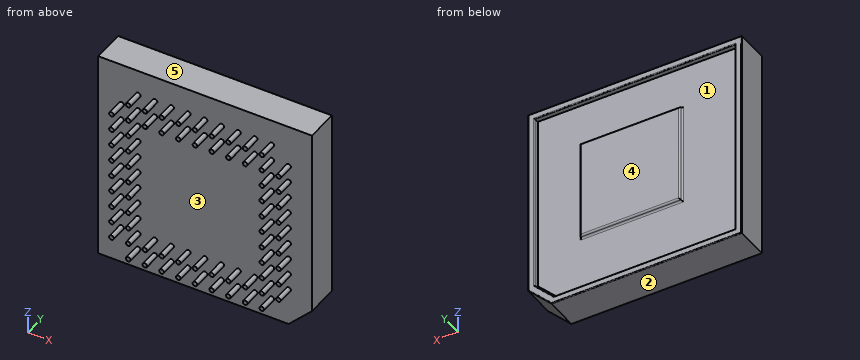
from build123d import *

# Parameters (mm, degrees)
BASE_EXTRUDE_DEPTH   = 5.08
CUT_EXTRUDE1_DEPTH   = 4.064
BOSS_EXTRUDE1_DEPTH  = 3.556
SKETCH4_W            = 15.24
SKETCH4_H            = 15.24
BOSS_EXTRUDE2_DEPTH  = 0.508
FILLET2_R            = 0.127
FILLET3_R            = 0.254
SKETCH5_R            = 0.3556
BOSS_EXTRUDE3_DEPTH  = 2.54
LPATTERN1_COUNT      = 10
LPATTERN1_PITCH      = 2.54
LPATTERN1_COUNT_DIR2 = 11
LPATTERN1_PITCH_DIR2 = 2.54
LPATTERN2_COUNT      = 2
LPATTERN2_PITCH      = 2.54
LPATTERN2_COUNT_DIR2 = 11
LPATTERN2_PITCH_DIR2 = 2.54


with BuildPart() as part:
    # Sketch1 → Base-Extrude (new body)
    with BuildSketch(Plane(origin=(0, 0, 0), x_dir=(1, 0, 0), z_dir=(0, 1, 0))):
        Polygon((0, 16.256), (3.556, 12.7), (3.556, -16.256), (-28.956, -16.256), (-28.956, 16.256), align=None)
    extrude(amount=BASE_EXTRUDE_DEPTH)

    # Sketch2 → Cut-Extrude1 (cut)
    with BuildSketch(Plane(origin=(0, 5.08, 0), x_dir=(-1, 0, 0), z_dir=(0, 1, 0))):
        Polygon((27.94, -15.24), (27.94, 15.24), (-2.54, 15.24), (-2.54, -12.279159021), (0.420840979, -15.24), align=None)
    extrude(amount=-CUT_EXTRUDE1_DEPTH, mode=Mode.SUBTRACT)

    # Sketch3 → Boss-Extrude1 (add)
    with BuildSketch(Plane(origin=(0, 1.016, 0), x_dir=(-1, 0, 0), z_dir=(0, 1, 0))):
        Polygon((0.526051224, -14.986), (27.686, -14.986), (27.686, 14.986), (-2.286, 14.986), (-2.286, -12.173948776), align=None)
    extrude(amount=BOSS_EXTRUDE1_DEPTH)

    # Sketch4 → Boss-Extrude2 (add)
    with BuildSketch(Plane(origin=(0, 4.572, 0), x_dir=(-1, 0, 0), z_dir=(0, 1, 0))):
        with Locations((11.971914099, 0.728085901)):
            Rectangle(SKETCH4_W, SKETCH4_H)
    extrude(amount=BOSS_EXTRUDE2_DEPTH)

    # Fillet2
    fillet2_edges = [part.edges().sort_by_distance(p)[0] for p in [
        (3.556, 5.08, 1.778),
        (1.778, 5.08, -14.478),
        (-14.478, 5.08, -16.256),
        (-14.18042049, 5.08, -15.24),
        (-27.94, 5.08, 0),
        (-12.7, 5.08, 15.24),
        (2.54, 5.08, 1.48042049),
        (1.05957951, 5.08, -13.75957951),
        (-28.956, 5.08, 0),
        (-12.7, 5.08, 16.256),
    ]]
    fillet(fillet2_edges, radius=FILLET2_R)

    # Fillet3
    fillet3_edges = [part.edges().sort_by_distance(p)[0] for p in [
        (-4.351914099, 4.572, 0.728085901),
        (-11.971914099, 4.572, -6.891914099),
        (-19.591914099, 4.572, 0.728085901),
        (-11.971914099, 4.572, 8.348085901),
        (-4.351914099, 5.08, 0.728085901),
        (-11.971914099, 5.08, -6.891914099),
        (-19.591914099, 5.08, 0.728085901),
        (-11.971914099, 5.08, 8.348085901),
    ]]
    fillet(fillet3_edges, radius=FILLET3_R - 0.0001)  # a hair under: the kernel refuses the full size

    # Sketch5 → Boss-Extrude3 (add)
    with BuildSketch(Plane.XZ):
        with Locations(Location((0, -10.541, 0), (0, 0, 90))):
            Circle(SKETCH5_R)
    boss_extrude3 = extrude(amount=BOSS_EXTRUDE3_DEPTH)

    # LPattern1: Boss-Extrude3 10 × 11, 51 skipped
    with Locations(*[(-j * LPATTERN1_PITCH_DIR2, 0, i * LPATTERN1_PITCH) for i in range(LPATTERN1_COUNT) for j in range(LPATTERN1_COUNT_DIR2) if (i, j) not in ((0, 0), (1, 2), (1, 3), (1, 4), (1, 5), (1, 6), (1, 7), (1, 8), (2, 2), (2, 3), (2, 4), (2, 5), (2, 6), (2, 7), (2, 8), (3, 2), (3, 3), (3, 4), (3, 5), (3, 6), (3, 7), (3, 8), (4, 2), (4, 3), (4, 4), (4, 5), (4, 6), (4, 7), (4, 8), (5, 2), (5, 3), (5, 4), (5, 5), (5, 6), (5, 7), (5, 8), (6, 2), (6, 3), (6, 4), (6, 5), (6, 6), (6, 7), (6, 8), (7, 2), (7, 3), (7, 4), (7, 5), (7, 6), (7, 7), (7, 8), (9, 0), (9, 10))]):
        add(boss_extrude3)

    # LPattern2: Boss-Extrude3 2 × 11, 2 skipped
    with Locations(*[(-j * LPATTERN2_PITCH_DIR2, 0, -i * LPATTERN2_PITCH) for i in range(LPATTERN2_COUNT) for j in range(LPATTERN2_COUNT_DIR2) if (i, j) not in ((0, 0), (1, 0), (1, 10))]):
        add(boss_extrude3)


solid = part.part
Build history of the part. All positions in model axes, mm. Face numbers are marked on the shaded views. A direction names the side the tool comes from. Give positions to 0.01 mm unless a question says otherwise; leave off trailing zeros. Order: outer loops, then holes, each group sorted by start corner. A loop starts at its lowest first (then second) coordinate and runs counter-clockwise, first axis right, second up. Notation, with made-up numbers: M -34,26.5 L 5,26.5 A21 cw 5,58.5 Z; hole C 79,37 d3. An arc over 180 degrees is marked long. Put each result on its own line as item: value.
Item 1: Slice it at D-D, the plane x = -24. Write the cut outline in (y, z).
From the geometry:
outline: M 0,-16.26 L 4.95,-16.26 A0.13 ccw 5.08,-16.13 L 5.08,-15.37 A0.13 ccw 4.95,-15.24 L 1.02,-15.24 L 1.02,-14.99 L 4.57,-14.99 L 4.57,14.99 L 1.02,14.99 L 1.02,15.24 L 4.95,15.24 A0.13 ccw 5.08,15.37 L 5.08,16.13 A0.13 ccw 4.95,16.26 L 0,16.26 Z
Item 2: 3-axis set-ups, long thin cutter, end or side, ignore diameter. For the marked faces 1 and 2: which of +Z, -Z, +X, -X, +Y, -Y reach the whole face in a straight line?
From the geometry:
face 1: +Y
face 2: -Z, +X, -X, +Y, -Y
Item 3: Two-plate mould, pull along Z, no slides. Class the marked faces 3, 4 and 5: +Z half, -Z half, draft (parallel to the pull), parting line (faces both ways), or undercut.
From the geometry:
face 3: undercut
face 4: draft
face 5: +Z half
Item 4: Slice it at A-A, the plane y = 2. Write the cut outline in (x, z).
From the geometry:
outline: M -28.96,-16.26 L 0,-16.26 L 3.56,-12.7 L 3.56,16.26 L -28.96,16.26 Z; M -27.69,-14.99 L -0.53,-14.99 L 2.29,-12.17 L 2.29,14.99 L -27.69,14.99 Z; hole M -27.94,-15.24 L -0.42,-15.24 L 2.54,-12.28 L 2.54,15.24 L -27.94,15.24 Z
Item 5: Flat gauge pin, fed straight in: pin 1 Ø1.5 at (x, z) = (-20.5, -8) entering from -Y. Where does the tip first touch, or does it go through?
From the geometry:
pin 1: stops at y = 0
Item 6: Probe line 1 (X direction, y = 2, z = 5); line 2 (Z direction, x = -14.5, y = 3); line 3 (X direction, y = -1.75, z = 5). List the from-to ranges inside material, lowest first. Write a range as [from, to].
From the geometry:
line 1: x = [-28.96, -27.94], [-27.69, 2.29], [2.54, 3.56]
line 2: z = [-16.26, -15.24], [-14.99, 14.99], [15.24, 16.26]
line 3: x = [-25.59, -25.21], [-23.05, -22.67], [-2.73, -2.35], [-0.19, 0.19]
